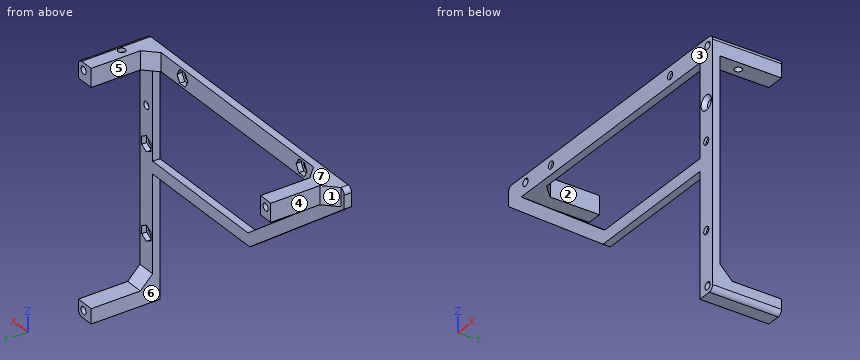
```python
from build123d import *

# Parameters (mm, degrees)
SKETCH1_R               = 1.5
BOSS_EXTRUDE1_DEPTH     = 3
SKETCH2_W               = 6
SKETCH2_H               = 7.5
BOSS_EXTRUDE2_DEPTH     = 25
CHAMFER3_SIZE           = 5
CHAMFER6_SIZE           = 5
CHAMFER8_SIZE           = 5
SKETCH3_R               = 1.5
CUT_EXTRUDE1_DEPTH      = 107.236732571
BOSS_EXTRUDE3_DEPTH     = 3
CUT_EXTRUDE2_DEPTH      = 2
CUT_EXTRUDE3_DEPTH      = 10
CUT_EXTRUDE3_DEPTH_BACK = 106.977560584
SKETCH6_R               = 1.5
SKETCH9_R               = 1.493282486
CUT_EXTRUDE4_DEPTH      = 10
CHAMFER9_SIZE           = 1.5


with BuildPart() as part:
    # Sketch1 → Boss-Extrude1 (new body)
    with BuildSketch(Plane(origin=(0, 0, 0), x_dir=(1, 0, 0), z_dir=(0, 1, 0))):
        with BuildLine():
            Line((40.047169811, 27.523584906), (44.547169811, 27.523584906))
            Line((44.547169811, 27.523584906), (45.547169811, 27.523584906))
            ThreePointArc((45.547169811, 27.523584906), (46.961383374, 26.937798468), (47.547169811, 25.523584906))
            Line((47.547169811, 25.523584906), (47.547169811, 24.523584906))
            Line((47.547169811, 24.523584906), (47.547169811, -70.476415094))
            ThreePointArc((47.547169811, -70.476415094), (46.961383374, -71.890628657), (45.547169811, -72.476415094))
            Line((45.547169811, -72.476415094), (-69.452830189, -72.476415094))
            Line((-69.452830189, -72.476415094), (-70.452830189, -72.476415094))
            ThreePointArc((-70.452830189, -72.476415094), (-71.867043751, -71.890628657), (-72.452830189, -70.476415094))
            Line((-72.452830189, -70.476415094), (-72.452830189, -69.476415094))
            Line((-72.452830189, -69.476415094), (-72.452830189, -64.976415094))
            Line((-72.452830189, -64.976415094), (40.047169811, -64.976415094))
            Line((40.047169811, -64.976415094), (40.047169811, 27.523584906))
        make_face()
        with Locations(Location((44.547169811, 24.523584906, 0), (0, 0, 270))):
            Circle(SKETCH1_R, mode=Mode.SUBTRACT)
        with Locations(Location((44.547169811, -69.476415094, 0), (0, 0, 270))):
            Circle(SKETCH1_R, mode=Mode.SUBTRACT)
        with Locations(Location((-62.452830189, -69.476415094, 0), (0, 0, 270))):
            Circle(SKETCH1_R, mode=Mode.SUBTRACT)
    extrude(amount=BOSS_EXTRUDE1_DEPTH)

    # Sketch2 → Boss-Extrude2 (add)
    with BuildSketch(Plane(origin=(0, 3, 0), x_dir=(1, 0, 0), z_dir=(0, 1, 0))):
        with BuildLine():
            Line((40.047169811, -64.976415094), (47.547169811, -64.976415094))
            Line((47.547169811, -64.976415094), (47.547169811, -70.476415094))
            ThreePointArc((47.547169811, -70.476415094), (46.961383374, -71.890628657), (45.547169811, -72.476415094))
            Line((45.547169811, -72.476415094), (40.047169811, -72.476415094))
            Line((40.047169811, -72.476415094), (40.047169811, -64.976415094))
        make_face()
        with Locations((-62.452830189, -68.726415094)):
            Rectangle(SKETCH2_W, SKETCH2_H)
        with BuildLine():
            Line((40.047169811, 21.523584906), (47.547169811, 21.523584906))
            Line((47.547169811, 21.523584906), (47.547169811, 25.523584906))
            ThreePointArc((47.547169811, 25.523584906), (46.961383374, 26.937798468), (45.547169811, 27.523584906))
            Line((45.547169811, 27.523584906), (40.047169811, 27.523584906))
            Line((40.047169811, 27.523584906), (40.047169811, 21.523584906))
        make_face()
    extrude(amount=BOSS_EXTRUDE2_DEPTH)

    # Chamfer3
    chamfer3_edges = [part.edges().sort_by_distance(p)[0] for p in [
        (43.797169811, 3, -21.523584906),
    ]]
    chamfer(chamfer3_edges, length=CHAMFER3_SIZE)

    # Chamfer6
    # the kernel refuses this chamfer: 5 mm, written as the material it adds along each edge
    with BuildSketch(Plane(origin=(40.047169811, 3, 72.476415094), x_dir=(0.027495876610586317, 0.9996219169112968, 0), z_dir=(0, 0, -1))) as chamfer6_piece_1:
        Polygon((CHAMFER6_SIZE * 0.999621916911, -CHAMFER6_SIZE * 0.0274958766106), (-CHAMFER6_SIZE * 0.0274958766106, -CHAMFER6_SIZE * 0.999621916911), (0, 0), align=None)
    extrude(amount=7.5)

    # Chamfer8
    chamfer8_edges = [part.edges().sort_by_distance(p)[0] for p in [
        (-65.452830189, 3, 68.726415094),
        (-59.452830189, 3, 68.726415094),
    ]]
    chamfer(chamfer8_edges, length=CHAMFER8_SIZE)

    # Sketch3 → Cut-Extrude1 (cut, through all)
    with BuildSketch(Plane(origin=(0, 0, 0), x_dir=(-1, 0, 0), z_dir=(0, -1, 0))):
        with Locations(Location((62.452830189, -69.476415094, 0), (0, 0, 90))):
            Circle(SKETCH3_R)
        with Locations(Location((-44.547169811, -69.476415094, 0), (0, 0, 90))):
            Circle(SKETCH3_R)
        with Locations(Location((-44.547169811, 24.523584906, 0), (0, 0, 90))):
            Circle(SKETCH3_R)
    extrude(amount=-CUT_EXTRUDE1_DEPTH, mode=Mode.SUBTRACT)

    # Sketch4 → Boss-Extrude3 (add)
    with BuildSketch(Plane(origin=(0, 0, 0), x_dir=(-1, 0, 0), z_dir=(0, -1, 0))):
        Polygon((-40.047169811, -22.476415094), (16.900565623, -22.476415094), (72.452830189, -64.976415094), (64.952830189, -64.976415094), (15.93612616, -27.476415094), (-40.047169811, -27.476415094), align=None)
    extrude(amount=-BOSS_EXTRUDE3_DEPTH)

    # Sketch5 → Cut-Extrude2 (cut)
    with BuildSketch(Plane(origin=(0, 3, 0), x_dir=(1, 0, 0), z_dir=(0, 1, 0))):
        Polygon((-44.277403708, -68.726415094), (-45.865116948, -65.976415094), (-49.040543429, -65.976415094), (-50.628256669, -68.726415094), (-49.040543429, -71.476415094), (-45.865116948, -71.476415094), align=None)
        Polygon((25.722596292, -68.726415094), (24.134883052, -65.976415094), (20.959456571, -65.976415094), (19.371743331, -68.726415094), (20.959456571, -71.476415094), (24.134883052, -71.476415094), align=None)
        Polygon((43.797169811, -0.651841575), (46.547169811, 0.935871665), (46.547169811, 4.111298146), (43.797169811, 5.699011386), (41.047169811, 4.111298146), (41.047169811, 0.935871665), align=None)
        Polygon((43.797169811, -35.651841575), (46.547169811, -34.064128335), (46.547169811, -30.888701854), (43.797169811, -29.300988614), (41.047169811, -30.888701854), (41.047169811, -34.064128335), align=None)
    extrude(amount=-CUT_EXTRUDE2_DEPTH, mode=Mode.SUBTRACT)

    # Sketch6 → Cut-Extrude3 (cut, two sides: drawn at the far end of the back side and taken through both)
    with BuildSketch(Plane(origin=(0, 1, 0), x_dir=(1, 0, 0), z_dir=(0, 1, 0)).offset(-CUT_EXTRUDE3_DEPTH_BACK)):
        with Locations(Location((43.797169811, 2.523584906, 0), (0, 0, 270))):
            Circle(SKETCH6_R)
        with Locations(Location((43.797169811, -32.476415094, 0), (0, 0, 270))):
            Circle(SKETCH6_R)
        with Locations(Location((22.547169811, -68.726415094, 0), (0, 0, 270))):
            Circle(SKETCH6_R)
        with Locations(Location((-47.452830189, -68.726415094, 0), (0, 0, 270))):
            Circle(SKETCH6_R)
        with Locations(Location((43.797169811, -47.476415094, 0), (0, 0, 270))):
            Circle(SKETCH6_R)
    extrude(amount=CUT_EXTRUDE3_DEPTH + CUT_EXTRUDE3_DEPTH_BACK, mode=Mode.SUBTRACT)

    # Sketch9 → Cut-Extrude4 (cut)
    with BuildSketch(Plane.XY.offset(72.476415094)):
        with Locations((43.797169811, 13)):
            Circle(SKETCH9_R)
    extrude(amount=-CUT_EXTRUDE4_DEPTH, mode=Mode.SUBTRACT)

    # Chamfer9
    chamfer9_edges = [part.edges().sort_by_distance(p)[0] for p in [
        (43.797169811, 0, 45.976415094),
    ]]
    chamfer(chamfer9_edges, length=CHAMFER9_SIZE)


solid = part.part
```
Work out the finished part from the listing and answer in its coordinate system (mm). Face numbers are marked on the shaded views. A direction names the side the tool comes from. Give positions to 0.01 mm unless a question says otherwise; leave off trailing zeros. Order: outer loops, then holes, each group sorted by start corner. A loop starts at its lowest first (then second) coordinate and runs counter-clockwise, first axis right, second up. Notation, with made-up numbers: (34, -31.5) -> (69, -31.5) arc R32 ccw to (69, -1.5) -> close; hole circle Ø7 at (46, 75). An arc over 180 degrees is marked (long way). Answer as CSV lines item,"result". Start each with the question number.
(1) Section D-D, the plane z = 19.5 is taken. Write down the section's boundary in (x, y).
(2) Which of the six approach directions +Z, -Z, +X, -X, +Y, -Y give full straight-line access (tool end or side, diameter ignored) to the marked faces 4, 5, 6 and 7?
(3) Consider line 1 along Y through (x, z) = (21.5, 24.5); line 2 along X through (y, z) = (2.25, 23). Determine where each line is inside the solid, lowest interval first.
(4) For a pull along X with two mould halves and no side action, classify the marked faces 1, 2 and 3 as released by +X, released by -X, zero draft, split by the parting line, or undercut.
(5) Section C-C, the plane y = 13 is taken. Write down the section's boundary in (x, z), plus the area to 3 significant figures.
(6) Each of these flat-tipped pins is pushed along its axis until it touches: pin 1 Ø3.5 at (x, z) = (22.55, 68.73) entering from +Y; pin 2 Ø1 at (y, z) = (2.5, -2) entering from -X; pin 3 Ø2.5 at (x, y) = (7.5, 1.5) entering from -Z; pin 4 Ø4 at (x, z) = (43.8, 32.48) entering from -Y. Where does it stop, or does it pass through?
(7) Section B-B, the plane x = -2.5 is taken. Write down the section's boundary in (y, z), plus the area to 3 significant figures.
(8) Section A-A, the plane y = 20 is taken. Write down the section's boundary in (x, z).
Entries:
1,outline,"(40.05, 0) -> (47.55, 0) -> (47.55, 3) -> (40.05, 3) -> close"
2,face 4,"+Z, -Z, -X, +Y"
2,face 5,"+Z, -Z, +Y"
2,face 6,"-Z, -X, +Y, -Y"
2,face 7,"+Z, +X, -X, +Y, -Y"
3,line 1,"0 to 3"
3,line 2,"-17.58 to 47.55"
4,face 1,"released by -X"
4,face 2,"undercut"
4,face 3,"zero draft"
5,outline,"(-65.45, 64.98) -> (-59.45, 64.98) -> (-59.45, 72.48) -> (-65.45, 72.48) -> close; (40.05, -27.52) -> (45.55, -27.52) arc R2 ccw to (47.55, -25.52) -> (47.55, -21.52) -> (40.05, -21.52) -> close; (40.05, 64.98) -> (42.3, 64.98) -> (42.3, 72.48) -> (40.05, 72.48) -> close; (45.29, 64.98) -> (47.55, 64.98) -> (47.55, 70.48) arc R2 ccw to (45.55, 72.48) -> (45.29, 72.48) -> (45.29, 70.78) arc R1.5 cw to (45.29, 68.17) -> close; hole circle Ø3 at (-62.45, 69.48); hole circle Ø3 at (44.55, -24.52)"
5,area,"107 mm²"
6,pin 1,"y = 1"
6,pin 2,"x = 40.05"
6,pin 3,"z = 22.48"
6,pin 4,"y = 0"
7,outline,"(0, 22.48) -> (3, 22.48) -> (3, 27.48) -> (0, 27.48) -> close; (0, 64.98) -> (3, 64.98) -> (3, 72.48) -> (0, 72.48) -> close"
7,area,"37.5 mm²"
8,outline,"(-65.45, 64.98) -> (-59.45, 64.98) -> (-59.45, 72.48) -> (-65.45, 72.48) -> close; (40.05, -27.52) -> (45.55, -27.52) arc R2 ccw to (47.55, -25.52) -> (47.55, -21.52) -> (40.05, -21.52) -> close; (40.05, 64.98) -> (47.55, 64.98) -> (47.55, 70.48) arc R2 ccw to (45.55, 72.48) -> (40.05, 72.48) -> close; hole circle Ø3 at (-62.45, 69.48); hole circle Ø3 at (44.55, -24.52); hole circle Ø3 at (44.55, 69.48)"
